Model file for the job. Use its own axes, mm. Give positions to 0.01 mm unless a question says otherwise; leave off trailing zeros. Loops run counter-clockwise (first coordinate to the right, second up) from the corner with the lowest first, then second, coordinate; pieces in that order, holes last. Notation, with made-up numbers: M -19.75,6.5 L 31.25,6.5 A23 ccw 31.25,44.5 Z; hole C -33,-9 d7. An arc over 180 degrees is marked long. Answer in a Markdown table with one row per item.
Solid Edge part; units mm, degrees
sketch "Sketch1" plane through (0, 0, 0) normal (0, 0, 1) x (1, 0, 0)
  line L0 (-20.8143, -25.5503) -> (-19.9719, 29.256)
  line L1 (-19.9719, 29.256) -> (21.029, 28.7357)
  line L2 (21.029, 28.7357) -> (20.3333, -26.0726)
  line L3 (20.3333, -26.0726) -> (-20.8143, -25.5503)
  circle A0 centre (-8.0875, 2.1558) radius 1.2785
  circle A1 centre (18.2006, -5.0169) radius 1.0663
  circle A2 centre (18.2006, 8.1625) radius 1.1789
  circle A3 centre (18.6409, -1.6077) radius 0.6174
  circle A4 centre (13.985, 1.7931) radius 1.3315
extrude "ExtrudedProtrusion_1" add sketch "Sketch1" along normal blind 1.524
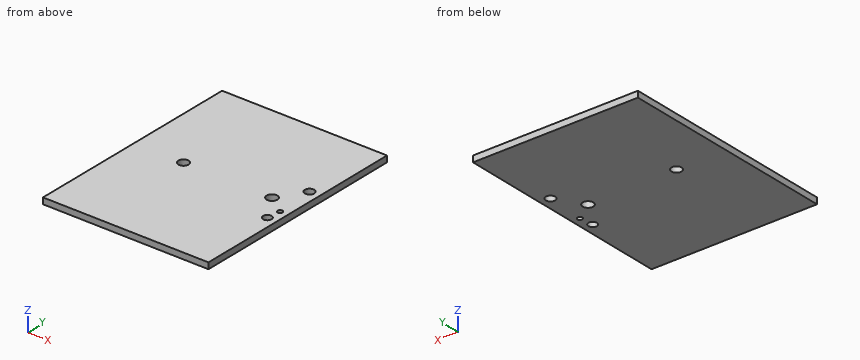
Q1. Drop flat-ended pins along their axis: pin 1 (1.4 mm diameter, centred on x = 18.64, y = -1.61, fed in from -Z); pin 2 (1.6 mm diameter, centred on x = 13.98, y = 1.79, fed in from +Z). Give the stop position or say it passes through.
Reported:
| item | result |
|---|---|
| pin 1 | z = 0 |
| pin 2 | through |
Q2. Saw through at C-C (y = 18.5). Give the cut face in (x, z).
Reported:
| item | result |
|---|---|
| outline | M -20.14,0 L 20.9,0 L 20.9,1.52 L -20.14,1.52 Z |
Q3. Saw through at D-D (y = -17). Give the cut face in (x, z), and give its area (3 significant figures).
Reported:
| item | result |
|---|---|
| outline | M -20.68,0 L 20.45,0 L 20.45,1.52 L -20.68,1.52 Z |
| area | 62.7 mm² |
Q4. Saw through at A-A (x = 14). Give the cut face in (y, z), and give its area (3 significant figures).
Reported:
| item | result |
|---|---|
| outline | M -25.99,0 L 0.46,0 L 0.46,1.52 L -25.99,1.52 Z; M 3.12,0 L 28.82,0 L 28.82,1.52 L 3.12,1.52 Z |
| area | 79.5 mm² |
Q5. Saw through at B-B (z = 0.65). Give the cut face in (x, y) (1 decimal), and give its area (3 significant figures).
Reported:
| item | result |
|---|---|
| outline | M -20.8,-25.6 L 20.3,-26.1 L 21,28.7 L -20,29.3 Z; hole C -8.1,2.2 d2.6; hole C 14,1.8 d2.7; hole C 18.2,8.2 d2.4; hole C 18.2,-5 d2.1; hole C 18.6,-1.6 d1.2 |
| area | 2,230 mm² |
Q6. Probe probe 1 along Y at (x, z) = (14.5, 1.4); probe 2 along Y at (x, z) = (13, 0.85); probe 3 along X at (y, z) = (-15, 0.85). List the from-to ranges inside material, lowest first.
Reported:
| item | result |
|---|---|
| probe 1 | -26 to 0.57, 3.02 to 28.82 |
| probe 2 | -25.98 to 0.9, 2.69 to 28.84 |
| probe 3 | -20.65 to 20.47 |
